Geometry: see drawing. Coordinates: mm, zero at the bounding-box minimum. Give positions to 0.01 mm unless a question says otherwise; leave off trailing zeros. Loops run counter-clockwise (first coordinate to the right, second up) from the corner with the lowest first, then second, coordinate; pieces in that order, holes last. Notation, with made-up numbers: (16.25, 62) -> (47.25, 62) arc R13 cw to (47.25, 67) -> close; hole circle Ø9 at (84.5, 51). An arc over 180 degrees is marked (long way). Return JSON: item names as keys, results as strings. Group by question number.
(1) Cut plane B-B on x = 1.05. Return loops of the section in (y, z), then the cut area to 3 significant figures.
(2) Cut plane D-D on y = 7. Return loops of the section in (x, z), then the cut area to 3 significant figures.
(3) Cut plane A-A on y = 20. Return loops of the section in (x, z).
(4) Cut plane C-C on z = 9. Return loops of the section in (x, y).
(5) Pin query (flat end, axial travel): pin 1 (1.5 mm diameter, centred on y = 25.5, z = 72.5, fed in from -X). Return the tip coordinate at first contact, or that it passes through.
(6) Ray query, line 1 (Y direction, x = 0.75, z = 10); line 2 (Y direction, x = 2, z = 98); line 3 (Y direction, x = 2.4, z = 102). Return the intervals inside material, ascending. Write a range as from..to.
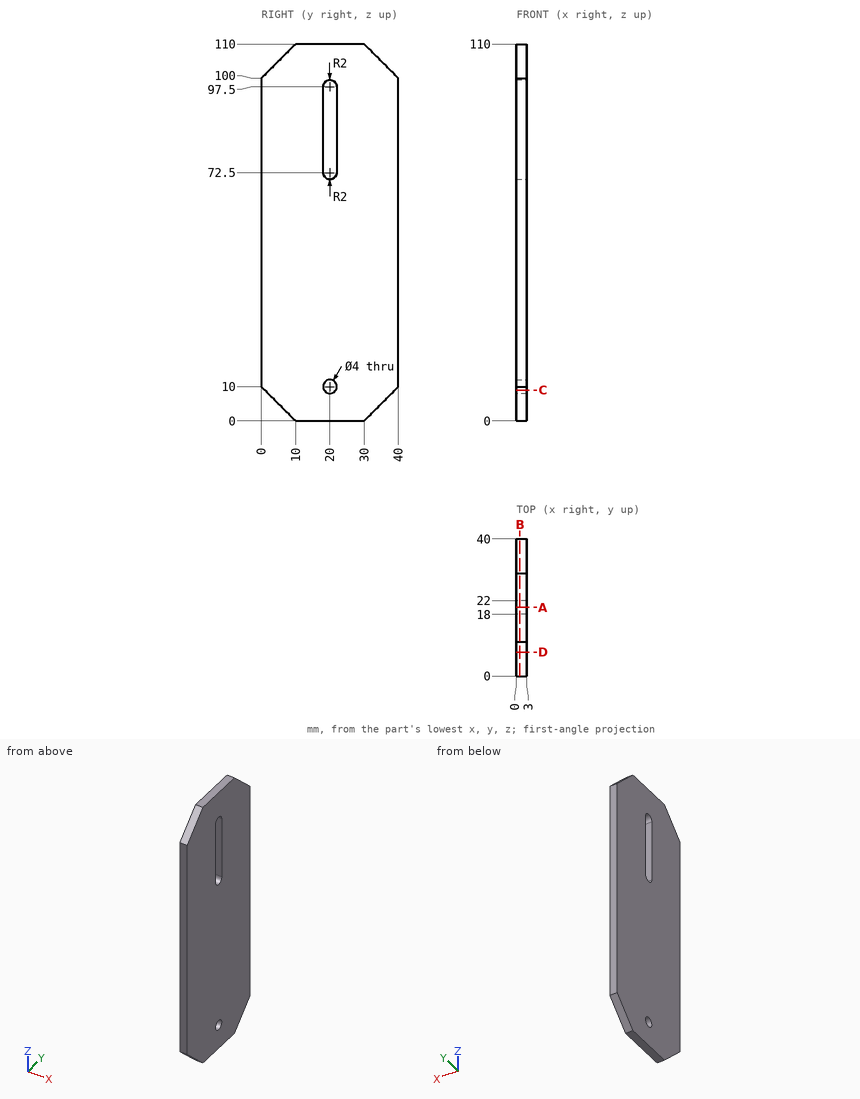
Answers:
{
 "1": {"outline": "(0, 10) -> (10, 0) -> (30, 0) -> (40, 10) -> (40, 100) -> (30, 110) -> (10, 110) -> (0, 100) -> close; hole circle Ø4 at (20, 10); hole (18, 72.5) arc R2 ccw to (22, 72.5) -> (22, 97.5) arc R2 ccw to (18, 97.5) -> close", "area": "4,070 mm²"},
 "2": {"outline": "(0, 3) -> (3, 3) -> (3, 107) -> (0, 107) -> close", "area": "312 mm²"},
 "3": {"outline": "(0, 0) -> (3, 0) -> (3, 8) -> (0, 8) -> close; (0, 12) -> (3, 12) -> (3, 70.5) -> (0, 70.5) -> close; (0, 99.5) -> (3, 99.5) -> (3, 110) -> (0, 110) -> close"},
 "4": {"outline": "(0, 1) -> (3, 1) -> (3, 18.27) -> (0, 18.27) -> close; (0, 21.73) -> (3, 21.73) -> (3, 39) -> (0, 39) -> close"},
 "5": {"pin 1": "x = 0"},
 "6": {"line 1": "0..18, 22..40", "line 2": "0..18.06, 21.94..40", "line 3": "2..38"}
}
